from build123d import *

# Parameters (mm, degrees)
SKETCH1_W           = 66
SKETCH1_H           = 72
SKETCH1_W_2         = 36
SKETCH1_H_2         = 40
BOSS_EXTRUDE1_DEPTH = 4
SKETCH2_R           = 2.5
CUT_EXTRUDE1_DEPTH  = 10
CUT_EXTRUDE3_DEPTH  = 10


with BuildPart() as part:
    # Sketch1 → Boss-Extrude1 (new body)
    with BuildSketch(Plane.XY):
        with Locations((33, 36)):
            Rectangle(SKETCH1_W, SKETCH1_H)
        with Locations((30, 36)):
            Rectangle(SKETCH1_W_2, SKETCH1_H_2, mode=Mode.SUBTRACT)
    extrude(amount=BOSS_EXTRUDE1_DEPTH)

    # Sketch2 → Cut-Extrude1 (cut)
    with BuildSketch(Plane.XY.offset(4)):
        with Locations((46.4, 63.5)):
            Circle(SKETCH2_R)
        with Locations((13.6, 63.5)):
            Circle(SKETCH2_R)
        with Locations((13.6, 10)):
            Circle(SKETCH2_R)
        with Locations((46.4, 10)):
            Circle(SKETCH2_R)
    extrude(amount=-CUT_EXTRUDE1_DEPTH, mode=Mode.SUBTRACT)

    # Sketch4 → Cut-Extrude3 (cut)
    with BuildSketch(Plane.XY.offset(4)):
        with BuildLine():
            Line((58, 46), (58, 26))
            ThreePointArc((58, 26), (56, 24), (54, 26))
            Line((54, 26), (54, 46))
            ThreePointArc((54, 46), (56, 48), (58, 46))
        make_face()
    extrude(amount=-CUT_EXTRUDE3_DEPTH, mode=Mode.SUBTRACT)


solid = part.part
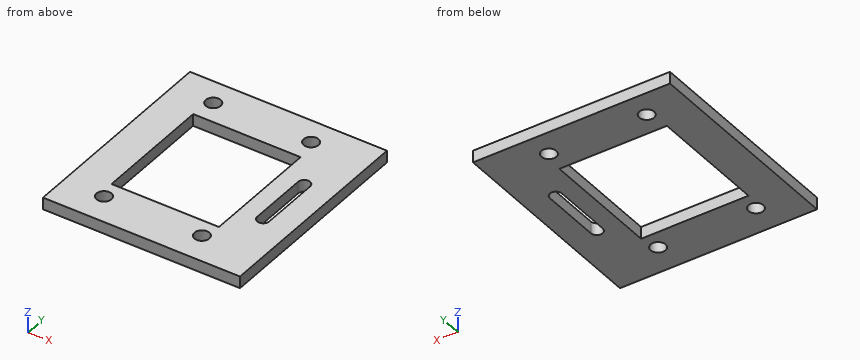
Can you work these out from the model? Positions are in its coordinate system, mm. Coordinates: 2 decimals unless noted, no trailing zeros. Write each loop counter-clockwise with the first axis right and the second up, starting at its lowest first coordinate (ties: lowest second). Pieces come first, ordered by that corner, then holes. Notation, with made-up numbers: (32.5, 78.5) -> (90.5, 78.5) arc R35 ccw to (90.5, 113.5) -> close; hole circle Ø9 at (-6.5, -37.75). An arc over 180 degrees is marked (long way). Write item = value, one per line.
(1) If I drill on probe 1 along Y at (x, z) = (13.6, 2.7); probe 2 along X at (y, z) = (46, 3.15); probe 3 along X at (y, z) = (53, 1.05), over which ranges is the centre line in solid material (lowest first)?
Verdict:
probe_1 = 0 to 7.5, 12.5 to 16, 56 to 61, 66 to 72
probe_2 = 0 to 12, 48 to 54, 58 to 66
probe_3 = 0 to 12, 48 to 66
(2) Imagine slicing it at A-A (y = 63.5). Please give me the cut outline in (x, z), and give its area (3 significant figures).
Verdict:
outline = (0, 0) -> (11.1, 0) -> (11.1, 4) -> (0, 4) -> close; (16.1, 0) -> (43.9, 0) -> (43.9, 4) -> (16.1, 4) -> close; (48.9, 0) -> (66, 0) -> (66, 4) -> (48.9, 4) -> close
area = 224 mm^2
(3) Imagine slicing it at C-C (z = 0.75). Please give me the cut outline in (x, y), and give its area (3 significant figures).
Verdict:
outline = (0, 0) -> (66, 0) -> (66, 72) -> (0, 72) -> close; hole circle Ø5 at (13.6, 10); hole circle Ø5 at (13.6, 63.5); hole (12, 16) -> (48, 16) -> (48, 56) -> (12, 56) -> close; hole circle Ø5 at (46.4, 10); hole circle Ø5 at (46.4, 63.5); hole (54, 26) arc R2 ccw to (58, 26) -> (58, 46) arc R2 ccw to (54, 46) -> close
area = 3,140 mm^2
(4) For pin 1 (1.2 mm diameter, centred on y = 26.5, z = 1.5, fed in from -X); pin 2 (4 mm diameter, centred on x = 46.4, y = 10, fed in from -Z), each with a flat end and sliding along its axis, tell me the tip position at first contact or that it passes through.
Verdict:
pin_1 = 0
pin_2 = through
(5) Imagine slicing it at B-B (x = 13.6). Please give me the cut outline in (y, z).
Verdict:
outline = (0, 0) -> (7.5, 0) -> (7.5, 4) -> (0, 4) -> close; (12.5, 0) -> (16, 0) -> (16, 4) -> (12.5, 4) -> close; (56, 0) -> (61, 0) -> (61, 4) -> (56, 4) -> close; (66, 0) -> (72, 0) -> (72, 4) -> (66, 4) -> close
(6) Imagine slicing it at D-D (y = 55). Please give me the cut outline in (x, z), and give its area (3 significant figures).
Verdict:
outline = (0, 0) -> (12, 0) -> (12, 4) -> (0, 4) -> close; (48, 0) -> (66, 0) -> (66, 4) -> (48, 4) -> close
area = 120 mm^2
